Autodesk Inventor part; units mm, degrees
ref_plane "YZ Plane" through (0, 0, 0) normal (1, 0, 0) x (0, 1, 0)
ref_plane "XZ Plane" through (0, 0, 0) normal (0, 1, 0) x (-1, 0, 0)
ref_plane "XY Plane" through (0, 0, 0) normal (0, 0, 1) x (1, 0, 0)
sketch "Sketch1" plane through (0, 0, 0) normal (0, 0, 1) x (1, 0, 0)
  line L0 (-759.3317, 185.2455) -> (256.6683, 185.2455)
  line L1 (-759.3317, -17.9545) -> (256.6683, -17.9545)
  line L2 (-759.3317, 185.2455) -> (-759.3317, 159.8455)
  line L3 (-759.3317, 159.8455) -> (-778.1277, 159.8455)
  line L4 (-778.1277, 159.8455) -> (-778.1277, 134.4455)
  line L5 (-778.1277, 134.4455) -> (-759.3317, 134.4455)
  line L6 (-759.3317, 134.4455) -> (-759.3317, 32.8455)
  line L7 (-759.3317, 32.8455) -> (-778.1277, 32.8455)
  line L8 (-778.1277, 32.8455) -> (-778.1277, 7.4455)
  line L9 (-778.1277, 7.4455) -> (-759.3317, 7.4455)
  line L10 (-759.3317, 7.4455) -> (-759.3317, -17.9545)
  line L11 (256.6683, 185.2455) -> (256.6683, 159.8455)
  line L12 (256.6683, 159.8455) -> (275.4643, 159.8455)
  line L13 (275.4643, 159.8455) -> (275.4643, 134.4455)
  line L14 (275.4643, 134.4455) -> (256.6683, 134.4455)
  line L15 (256.6683, 134.4455) -> (256.6683, 32.8455)
  line L16 (256.6683, 32.8455) -> (275.4643, 32.8455)
  line L17 (275.4643, 32.8455) -> (275.4643, 7.4455)
  line L18 (275.4643, 7.4455) -> (256.6683, 7.4455)
  line L19 (256.6683, 7.4455) -> (256.6683, -17.9545)
  point P0 (0, 0)
  dimension "d0" = 1016
  dimension "d1" = 203.2
  dimension "d2" = 25.4
  dimension "d3" = 25.4
  dimension "d4" = 25.4
  dimension "d5" = 25.4
  dimension "d6" = 18.796
  dimension "d7" = 18.796
  dimension "d8" = 18.796
  dimension "d9" = 25.4
  dimension "d11" = 25.4
  dimension "d12" = 25.4
  dimension "d15" = 25.4
extrude "Extrusion1" add sketch "Sketch1" along normal blind 18.796
sketch "Sketch2" plane through (0, 0, 18.796) normal (0, 0, 1) x (1, 0, 0)
  line L0 (-778.1277, 159.8455) -> (-759.3317, 159.8455)
  line L1 (275.4643, 159.8455) -> (256.6683, 159.8455)
  point P0 (0, 0)
  point P1 (-759.3317, 134.5414)
  point P2 (-759.3317, 32.5902)
  point P3 (-759.3317, 7.3202)
  point P4 (256.6683, 134.5414)
  point P5 (256.6683, 32.5902)
  point P6 (256.6683, 7.3202)
hole "Hole1" at (-759.3317, 159.8455, 18.796) at (-759.3317, 134.5414, 18.796) at (-759.3317, 32.5902, 18.796) at (-759.3317, 7.3202, 18.796) at (256.6683, 159.8455, 18.796) at (256.6683, 134.5414, 18.796) at (256.6683, 32.5902, 18.796) at (256.6683, 7.3202, 18.796) direction (0, 0, -1) diameter 6.35 end through all
sketch "Sketch3" plane through (0, 0, 18.796) normal (0, 0, 1) x (1, 0, 0)
  line L0 (-778.1277, 159.8455) -> (-778.1277, 134.4455)
  line L1 (-778.1277, 32.8455) -> (-778.1277, 7.4455)
  line L2 (-762.4964, 32.8455) -> (-778.1277, 32.8455)
  line L3 (-778.1277, 134.4455) -> (-762.5052, 134.4455)
  line L4 (275.4643, 159.8455) -> (275.4643, 134.4455)
  line L5 (275.4643, 159.8455) -> (259.8433, 159.8455)
  line L6 (275.4643, 32.8455) -> (259.833, 32.8455)
  line L7 (275.4643, 32.8455) -> (275.4643, 7.4455)
  point P0 (0, 0)
  point P1 (266.0663, 147.1455)
  point P2 (266.0663, 20.1455)
  point P3 (-768.7297, 20.1455)
  point P4 (-768.7297, 147.1455)
  dimension "d25" = 9.398
  dimension "d26" = 9.398
  dimension "d27" = 12.7
  dimension "d28" = 12.7
  dimension "d29" = 9.398
  dimension "d30" = 12.7
  dimension "d31" = 12.7
  dimension "d32" = 9.398
hole "Hole2" at (266.0663, 147.1455, 18.796) at (266.0663, 20.1455, 18.796) at (-768.7297, 20.1455, 18.796) at (-768.7297, 147.1455, 18.796) direction (0, 0, -1) diameter 6.35 end through all
sketch "Sketch4" plane through (0, 0, 18.796) normal (0, 0, 1) x (1, 0, 0)
  line L0 (-759.3317, 185.2455) -> (256.6683, 185.2455)
  line L1 (-251.3317, 185.2455) -> (-251.3317, -17.9545)
  line L2 (256.6683, -17.9545) -> (-759.3317, -17.9545)
  line L3 (-260.7297, 185.2455) -> (-260.7297, -17.9545)
  line L4 (-241.9337, 185.2455) -> (-241.9337, -17.9545)
  line L5 (-260.7297, 185.2455) -> (-241.9337, 185.2455)
  line L6 (-260.7297, -17.9545) -> (-241.9337, -17.9545)
  point P0 (0, 0)
  dimension "d40" = 9.398
  dimension "d41" = 9.398
extrude "Extrusion2" cut sketch "Sketch4" against normal blind 9.398
properties part number "shelf" material "Wood (Birch)"
The model under review builds one solid part; all positions refer to its coordinate system, in mm. A direction names the side the tool comes from. Round coordinates to 2 decimals unless told otherwise and drop trailing zeros. Order: outer loops, then holes, each group sorted by start corner. A loop starts at its lowest first (then second) coordinate and runs counter-clockwise, first axis right, second up.
(1) Wall thickness on L1, parallel to X at y = 135, z = 17.5; L2, parallel to X at y = 175, z = 15.5; L3, parallel to X at y = 29, z = 17.5: over which ranges is each line inside the solid? List them lowest first.
Working result:
L1: x = -778.13 to -762.47, -756.19 to -260.73, -241.93 to 253.53, 259.81 to 275.46
L2: x = -759.33 to -260.73, -241.93 to 256.67
L3: x = -778.13 to -260.73, -241.93 to 275.46
(2) For P1, Ø1, axis at y = 41.5, z = 4, coming from the +X side; P2, Ø5, axis at x = -759.33, y = 134.54, coming from the +Z side; P3, Ø5, axis at x = 146, y = 34, coming from the -Z side; P4, Ø8, axis at x = 265, z = 10, coming from the +Y side, all flat-tipped, find the tip position at first contact; note any pin that passes through.
Working result:
P1: stops at x = 256.67
P2: passes through
P3: stops at z = 0
P4: stops at y = 159.85
(3) Take a section at A-A, the plane y = 48. State the section outline as (x, z) points.
Working result:
outline: (-759.33, 0) - (256.67, 0) - (256.67, 18.8) - (-241.93, 18.8) - (-241.93, 9.4) - (-260.73, 9.4) - (-260.73, 18.8) - (-759.33, 18.8) - close
(4) Take a section at B-B, the plane z = 5.25. Count the separate pieces of the cut face and the enclosed holes in it, plus the area to 3 significant figures.
Working result:
separate pieces: 1
enclosed holes: 4
area: 208,000 mm2
(5) Mouldability with a two-part tool opening along X and no side actions: class faces 4 (the face through (-251, 85, 9.398)), 5 (the face through (256.668, 84, 9)), 6 (the face through (-258, -17.954, 9)) as released by +X, released by -X, zero draft, split by the parting line, or undercut.
Working result:
face 4: undercut
face 5: released by +X
face 6: zero draft
(6) Tool access review of faces 1 (the face through (-759.332, 174, 9)), 2 (the face through (256.668, -7, 9)), 3 (the face through (-759.332, 84, 9)): name each direction out of +Z, -Z, +X, -X, +Y, -Y from which nothing blocks a thin tool from reaching the whole face with its end or side.
Working result:
face 1: +Z, -Z, -X, +Y
face 2: +Z, -Z, +X, -Y
face 3: +Z, -Z, -X
